Answer from the drawing. Dimensions are ordinates in mm from the lowest x, y and z of the part. Give positions to 0.01 mm unless a question says otherwise; leave off trailing zeros. Loops run counter-clockwise (first coordinate to the right, second up) from the corner with the lowest first, then second, coordinate; pieces in that order, holes last. Notation, with made-up numbers: (-36, 8) - (-8, 8) arc R7 ccw to (-8, 20) - close; hole circle Ø2 at (80.25, -3.5). An arc over 180 degrees is marked (long way). Put each result on its own line as item: value. Start each with the question number.
1. Consider L1, parallel to Z at x = 47.5, y = 1.45; L2, parallel to X at y = 2.85, z = 16.5; L3, parallel to X at y = 2.2, z = 80. Determine where each line is inside the solid, lowest interval first. Write a range as from..to.
2. A cutting plane is placed at B-B, the plane z = 47.5. Determine the outline of the cut face in (x, y), plus the area to 3 significant figures.
3. A cutting plane is placed at D-D, the plane z = 74.5. Determine the outline of the cut face in (x, y).
4. A cutting plane is placed at C-C, the plane x = 17. Determine the outline of the cut face in (y, z).
5. A cutting plane is placed at A-A, the plane y = 1.45. Count the separate pieces of the cut face and the enclosed holes in it, plus the area to 3 significant figures.
6. Given pin 1 Ø1.5 at (x, y) = (52, 1) entering from +Z; pin 2 Ø1.5 at (y, z) = (2, 16.5) entering from +X; pin 3 Ø1.5 at (y, z) = (2, 16.5) entering from -X; pin 4 Ø1.8 at (x, z) = (47.5, 39.5) entering from -Y, each flat-ended and moving along its own axis, determine where each tip first touches the part or whether it passes through.
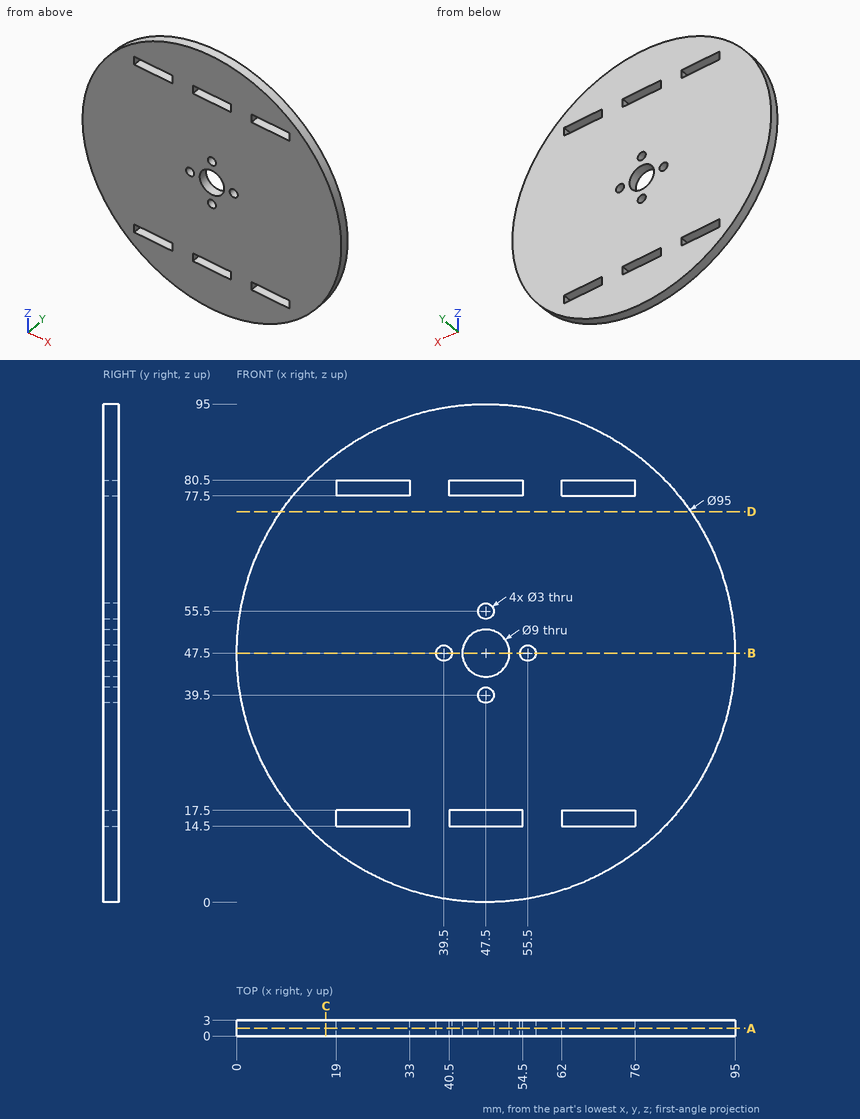
Return value:
1. L1: z = 0..14.5, 17.5..38, 41..43, 52..54, 57..77.5, 80.5..95
1. L2: x = 11.51..19, 33..40.5, 54.5..62, 76..83.49
1. L3: x = 12.86..19, 33..40.5, 54.5..62, 76..82.14
2. outline: (0, 0) - (38, 0) - (38, 3) - (0, 3) - close; (41, 0) - (43, 0) - (43, 3) - (41, 3) - close; (52, 0) - (54, 0) - (54, 3) - (52, 3) - close; (57, 0) - (95, 0) - (95, 3) - (57, 3) - close
2. area: 240 mm2
3. outline: (8.42, 0) - (86.58, 0) - (86.58, 3) - (8.42, 3) - close
4. outline: (0, 11.09) - (3, 11.09) - (3, 83.91) - (0, 83.91) - close
5. separate pieces: 1
5. enclosed holes: 11
5. area: 6,740 mm2
6. pin 1: stops at z = 94.85
6. pin 2: stops at x = 84.12
6. pin 3: stops at x = 10.88
6. pin 4: passes through
